```python
from build123d import *

# Parameters (mm, degrees)
SKETCH_1_W          = 37
SKETCH_1_H          = 30
SKETCH_1_W_2        = 10.3
SKETCH_1_H_2        = 10.3
EXTRUDE_1_DEPTH     = 30
SKETCH_2_R          = 1.65
SKETCH_2_W          = 11.25
SKETCH_2_H          = 10
CUT_EXTRUDE_1_DEPTH = 39.304699451
SKETCH_3_R          = 5
SKETCH_3_W          = 15.85
SKETCH_3_H          = 3.119518618
CUT_EXTRUDE_2_DEPTH = 39.304699451
SKETCH_4_W          = 18
SKETCH_4_H          = 14.880481382
CUT_EXTRUDE_3_DEPTH = 50.939963957
SKETCH_5_W          = 5.85
SKETCH_5_H          = 4.85
EXTRUDE_2_DEPTH     = 18
FILLET_2_R          = 3.12


with BuildPart() as part:
    # 草图1 → 凸台-拉伸1 (new body)
    with BuildSketch(Plane.XY):
        Rectangle(SKETCH_1_W, SKETCH_1_H)
        with Locations((7.5, 5)):
            Rectangle(SKETCH_1_W_2, SKETCH_1_H_2, mode=Mode.SUBTRACT)
    extrude(amount=EXTRUDE_1_DEPTH)

    # 草图2 → 切除-拉伸1 (cut, through all)
    with BuildSketch(Plane.XY.offset(30)):
        with Locations((-13.75, 5.880481382)):
            Circle(SKETCH_2_R)
        with Locations((-13.75, -10.119518618)):
            Circle(SKETCH_2_R)
        with Locations((1.25, -10.119518618)):
            Circle(SKETCH_2_R)
        with Locations((12.875, -10)):
            Rectangle(SKETCH_2_W, SKETCH_2_H)
    extrude(amount=-CUT_EXTRUDE_1_DEPTH, mode=Mode.SUBTRACT)

    # 草图3 → 切除-拉伸2 (cut, through all)
    with BuildSketch(Plane.XY.offset(30)):
        with Locations((-6.25, -2.119518618)):
            Circle(SKETCH_3_R)
        with Locations((-10.575, 13.440240691)):
            Rectangle(SKETCH_3_W, SKETCH_3_H)
    extrude(amount=-CUT_EXTRUDE_2_DEPTH, mode=Mode.SUBTRACT)

    # 草图4 → 切除-拉伸3 (cut, through all)
    with BuildSketch(Plane.ZY.offset(18.5)):
        with Locations((15, -1.559759309)):
            Rectangle(SKETCH_4_W, SKETCH_4_H)
    extrude(amount=-CUT_EXTRUDE_3_DEPTH, mode=Mode.SUBTRACT)

    # 草图5 → 凸台-拉伸2 (add)
    with BuildSketch(Plane.XY.offset(6)):
        with Locations((15.575, -2.575)):
            Rectangle(SKETCH_5_W, SKETCH_5_H)
    extrude(amount=EXTRUDE_2_DEPTH)

    # 圆角2
    # the kernel refuses this fillet: 3.12 mm, written as the material it adds along each edge
    with BuildSketch(Plane(origin=(7.25, -5, 6), x_dir=(0, -1, 0), z_dir=(0, 0, -1)), Plane(origin=(7.25, -5, 30), x_dir=(0, -1, 0), z_dir=(0, 0, -1))) as fillet_2_piece_1:
        with BuildLine():
            CenterArc((FILLET_2_R, -FILLET_2_R), FILLET_2_R, 90, 90)
            Line((0, -FILLET_2_R), (-FILLET_2_R * 0.02, -FILLET_2_R))
            Line((-FILLET_2_R * 0.02, -FILLET_2_R), (-FILLET_2_R * 0.02, FILLET_2_R * 0.02))
            Line((-FILLET_2_R * 0.02, FILLET_2_R * 0.02), (FILLET_2_R, FILLET_2_R * 0.02))
            Line((FILLET_2_R, FILLET_2_R * 0.02), (FILLET_2_R, 0))
        make_face()
    extrude(amount=6)
    with BuildSketch(Plane(origin=(-2.65, 11.880481382, 30), x_dir=(0, 1, 0), z_dir=(0, 0, -1))) as fillet_2_piece_2:
        with BuildLine():
            CenterArc((FILLET_2_R, -FILLET_2_R), FILLET_2_R, 90, 90)
            Line((0, -FILLET_2_R), (-FILLET_2_R * 0.02, -FILLET_2_R))
            Line((-FILLET_2_R * 0.02, -FILLET_2_R), (-FILLET_2_R * 0.02, FILLET_2_R * 0.02))
            Line((-FILLET_2_R * 0.02, FILLET_2_R * 0.02), (FILLET_2_R, FILLET_2_R * 0.02))
            Line((FILLET_2_R, FILLET_2_R * 0.02), (FILLET_2_R, 0))
        make_face()
    extrude(amount=30)
    # the kernel refuses this fillet: 3.12 mm, written as the material it takes off along each edge
    with BuildSketch(Plane(origin=(-18.5, 11.880481382, 30), x_dir=(1, 0, 0), z_dir=(0, 0, -1)), Plane(origin=(18.5, -5, 30), x_dir=(-1, 0, 0), z_dir=(0, 0, -1)), Plane(origin=(7.25, -15, 30), x_dir=(-1, 0, 0), z_dir=(0, 0, -1))) as fillet_2_2_piece_1:
        with BuildLine():
            CenterArc((FILLET_2_R, FILLET_2_R), FILLET_2_R, 180, 90)
            Line((0, FILLET_2_R), (-FILLET_2_R * 0.02, FILLET_2_R))
            Line((-FILLET_2_R * 0.02, FILLET_2_R), (-FILLET_2_R * 0.02, -FILLET_2_R * 0.02))
            Line((-FILLET_2_R * 0.02, -FILLET_2_R * 0.02), (FILLET_2_R, -FILLET_2_R * 0.02))
            Line((FILLET_2_R, -FILLET_2_R * 0.02), (FILLET_2_R, 0))
        make_face()
    extrude(amount=30, mode=Mode.SUBTRACT)
    with BuildSketch(Plane(origin=(18.5, 15, 0), x_dir=(0, -1, 0), z_dir=(0, 0, 1)), Plane(origin=(-18.5, -15, 0), x_dir=(0, 1, 0), z_dir=(0, 0, 1))) as fillet_2_2_piece_2:
        with BuildLine():
            CenterArc((FILLET_2_R, -FILLET_2_R), FILLET_2_R, 90, 90)
            Line((0, -FILLET_2_R), (-FILLET_2_R * 0.02, -FILLET_2_R))
            Line((-FILLET_2_R * 0.02, -FILLET_2_R), (-FILLET_2_R * 0.02, FILLET_2_R * 0.02))
            Line((-FILLET_2_R * 0.02, FILLET_2_R * 0.02), (FILLET_2_R, FILLET_2_R * 0.02))
            Line((FILLET_2_R, FILLET_2_R * 0.02), (FILLET_2_R, 0))
        make_face()
    extrude(amount=30, mode=Mode.SUBTRACT)


solid = part.part
```
The listing builds one solid part. Answer for the finished solid, in the listing's coordinates (mm). A direction names the side the tool comes from. Give positions to 0.01 mm unless a question says otherwise; leave off trailing zeros. Order: outer loops, then holes, each group sorted by start corner. A loop starts at its lowest first (then second) coordinate and runs counter-clockwise, first axis right, second up.
1) Find section C-C on x = 14. Write down the section's boundary in (y, z), then the cut area to 3 significant figures.
Reported:
outline: (-5, 0) - (15, 0) - (15, 30) - (-5, 30) - close; hole (-0.15, 6) - (5.88, 6) - (5.88, 24) - (-0.15, 24) - close
area: 491 mm2
2) For faces 1 (the face through (-3.54, 12.82, 15.21)), 2 (the face through (17.61, 14.06, 14.79)), 3 (the face through (16, 3, 24)), 4 (the face through (7.25, -10, 15)), 5 (the face through (2.35, 6.1, 14.8)), determine the directions among +Z, -Z, +X, -X, +Y, -Y from which every point of the face is accessible in a straight line to the end or side of a thin tool.
Reported:
face 1: +Z, -Z, -X, +Y
face 2: +Z, -Z, +X, +Y
face 3: +X, -X
face 4: +Z, -Z, +X, -Y
face 5: +Z, -Z
3) Find section D-D on x = -13. Write down the section's boundary in (y, z), then the cut area to 3 significant figures.
Reported:
outline: (-15, 0) - (-11.59, 0) - (-11.59, 30) - (-15, 30) - close; (-8.65, 0) - (4.41, 0) - (4.41, 6) - (-8.65, 6) - close; (-8.65, 24) - (4.41, 24) - (4.41, 30) - (-8.65, 30) - close; (7.35, 0) - (11.88, 0) - (11.88, 30) - (7.35, 30) - close
area: 395 mm2
4) Given P1, Ø4.5, axis at x = 1.25, y = -10.12, coming from the +Z side; P2, Ø4, axis at y = -1.5, z = 10.5, coming from the -X side; P3, Ø9, axis at x = -6.25, y = -2.12, coming from the -Z side; P4, Ø0.9, axis at x = -16.5, z = 12.5, coming from the -Y side, each flat-ended and moving along its own axis, determine where each tip first touches the part or whether it passes through.
Reported:
P1: stops at z = 30
P2: stops at x = 12.65
P3: passes through
P4: stops at y = -14.93
5) Find section A-A on x = 1.25. Write down the section's boundary in (y, z), then the cut area to 3 significant figures.
Reported:
outline: (-15, 0) - (-11.77, 0) - (-11.77, 30) - (-15, 30) - close; (-8.47, 0) - (15, 0) - (15, 30) - (-8.47, 30) - (-8.47, 24) - (5.88, 24) - (5.88, 6) - (-8.47, 6) - close
area: 543 mm2
6) Find section B-B on z = 12.75. Give the number of separate pieces and of enclosed holes in the cut face, then the cut area to 3 significant figures.
Reported:
separate pieces: 3
enclosed holes: 0
area: 399 mm2
7) Consider line 1 along Z through (x, y) = (-10.5, 2); line 2 along Y through (x, z) = (1.25, 11.5); line 3 along Y through (x, z) = (-6.25, 1.9). Determine where each line is inside the solid, lowest interval first.
Reported:
line 1: z = 0 to 6, 24 to 30
line 2: y = -15 to -11.77, 5.88 to 15
line 3: y = -15 to -7.12, 2.88 to 11.88
8) Determine the mould class of faces 6 (the face through (0, 0, 0)), 7 (the face through (-13.965, 7.516, 15.21)), 8 (the face through (-17, 5.88, 15)) for opening direction Z: pulls with the +Z half, pulls with the -Z half, needs draft (parallel to the pull), parting line crosses it, or undercut.
Reported:
face 6: pulls with the -Z half
face 7: needs draft
face 8: undercut
